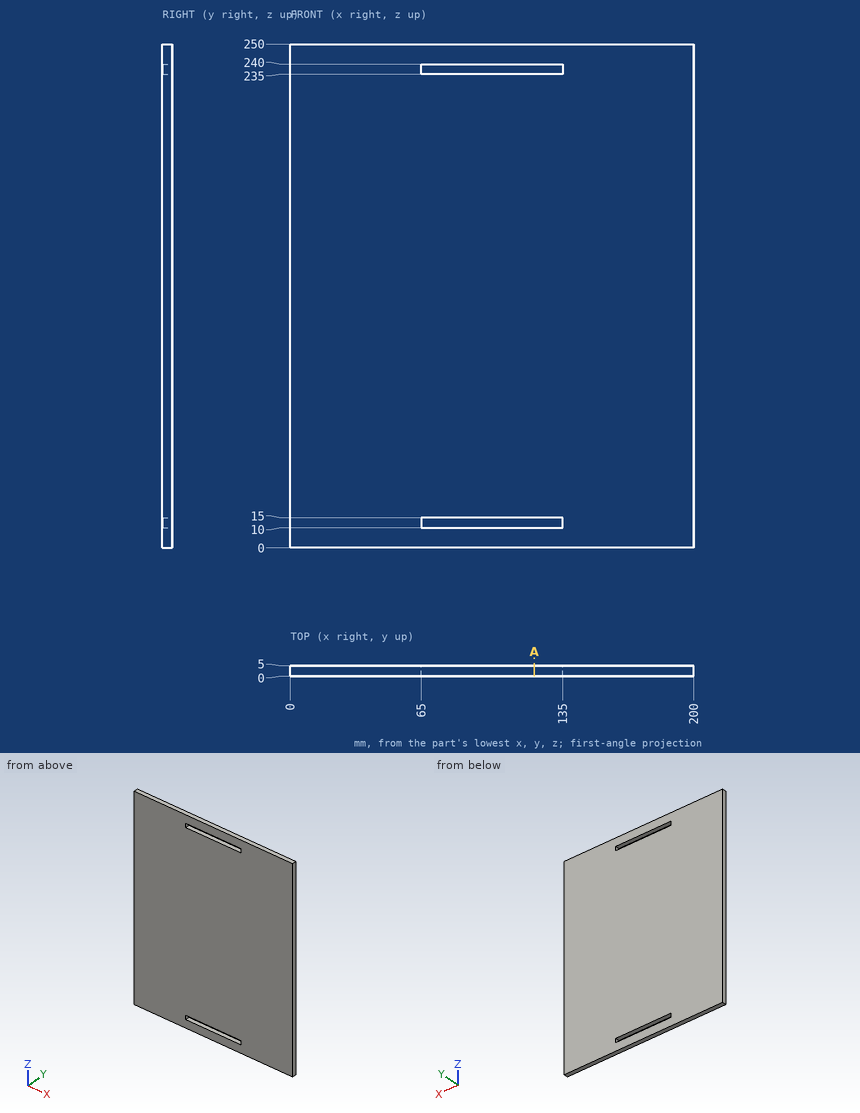
Verification items for this drawing (mm, ordinates from the low corner). Round coordinates to 2 decimals unless told otherwise and drop trailing zeros. Loops run counter-clockwise (first coordinate to the right, second up) from the corner with the lowest first, then second, coordinate; pieces in that order, holes last. Notation, with made-up numbers: (68.25, 41.25) -> (109.25, 41.25) arc R26 ccw to (109.25, 79.25) -> close; hole circle Ø1 at (21, 89). An arc over 180 degrees is marked (long way). Answer in a Markdown table with one row per item.
Q1. Go/stop test with a flat-tipped pin: P1, Ø8, axis at x = 55, z = 215.5, coming from the -Y side. Record where the tip stops, or that it passes through.
Data:
| item | result |
|---|---|
| P1 | stops at y = 0 |
Q2. Sectioned sample at A-A on x = 121. Enter the section's corners in (y, z), then the cut area to 3 significant figures.
Data:
| item | result |
|---|---|
| outline | (0, 0) -> (5, 0) -> (5, 10) -> (0, 10) -> close; (0, 15) -> (5, 15) -> (5, 235) -> (0, 235) -> close; (0, 240) -> (5, 240) -> (5, 250) -> (0, 250) -> close |
| area | 1,200 mm^2 |
Q3. Thickness scan on L1, parallel to Z at x = 100, y = 0.55; L2, parallel to X at y = 2, z = 237. Record the ranges inside material, lowest first.
Data:
| item | result |
|---|---|
| L1 | z = 0 to 10, 15 to 235, 240 to 250 |
| L2 | x = 0 to 65, 135 to 200 |
